```python
from build123d import *

# Parameters (mm, degrees)
F1_DEPTH = 26


with BuildPart() as f1:
    # F0 (on Top) → F1 (new body)
    with BuildSketch(Plane.XY):
        with BuildLine():
            ThreePointArc((-16.324504, 1), (-16.03161, 0.292893), (-15.324504, 0))
            Line((-15.324504, 0), (-0.324504, 0))
            ThreePointArc((-0.324504, 0), (0.382603, 0.292893), (0.675496, 1))
            ThreePointArc((0.675496, 1), (0.382603, 1.707107), (-0.324504, 2))
            Line((-0.324504, 2), (-13.324504, 2))
            ThreePointArc((-13.324504, 2), (-14.03161, 2.292893), (-14.324504, 3))
            Line((-14.324504, 3), (-14.324504, 8.393347))
            ThreePointArc((-14.324504, 8.393347), (-13.252645, 9.390761), (-12.334831, 8.25))
            Line((-12.334831, 8.25), (-0.564496, 8.25))
            Line((-0.564496, 8.25), (-0.564496, 8.948101))
            Line((-0.564496, 8.948101), (-0.564496, 9.25))
            ThreePointArc((-0.564496, 9.25), (-0.857389, 9.957107), (-1.564496, 10.25))
            Line((-1.564496, 10.25), (-15.324504, 10.25))
            ThreePointArc((-15.324504, 10.25), (-16.03161, 9.957107), (-16.324504, 9.25))
            Line((-16.324504, 9.25), (-16.324504, 1))
        make_face()
        with BuildLine():
            ThreePointArc((-12.334831, 8.25), (-13.252645, 9.390761), (-14.324504, 8.393347))
            Line((-14.324504, 8.393347), (-12.334831, 8.25))
        make_face()
    extrude(amount=F1_DEPTH)


solid = f1.part
```
Can you work these out from the model? Positions are in its coordinate system, mm. A direction names the side the tool comes from. Round coordinates to 2 decimals unless told otherwise and drop trailing zeros. Loops run counter-clockwise (first coordinate to the right, second up) from the corner with the lowest first, then second, coordinate; pieces in that order, holes last. Notation, with made-up numbers: (3.5, 24.5) -> (7.5, 24.5) arc R31 ccw to (7.5, 53.5) -> close; hole circle Ø1 at (45, 79). An arc over 180 degrees is marked (long way). One line per item, written item: value. Start each with the question number.
1. If we section it at D-D, the plane y = 6.5: Write out the boundary of the cut face in (x, z), then the cut area to 3 significant figures.
2. If we section it at A-A, the plane x = -12: Write out the boundary of the cut face in (y, z), then the cut area to 3 significant figures.
3. For pin 1 (1 mm diameter, centred on x = -13.5, y = 9, fed in from -Z); pin 2 (1.1 mm diameter, centred on y = 8.5, z = 15, fed in from +X); pin 3 (2.5 mm diameter, centred on y = 4.5, z = 18.5, fed in from +X), each with a flat end and sliding along its axis, tell me the tip position at first contact or that it passes through.
4. If we section it at C-C, the plane x = -1.25: Write out the boundary of the cut face in (y, z).
5. If I drill on probe 1 along Y at (x, z) = (-7, 17); probe 2 along X at (y, z) = (5, 24); probe 3 along Y at (x, z) = (-12.5, 6.75), over which ranges is the centre line in solid material (lowest first)?
6. If we section it at B-B, the plane z = 22.25: Write out the boundary of the cut face in (x, y).
7. For faces 1 (the flat face through (-7, 8.25, 13)), 2 (the cylindrical face through (-0.85, 9.95, 12.82)), 3 (the flat face through (-13.344, 8.323, 12.818)), which set-ups out of +Z, -Z, +X, -X, +Y, -Y let a thin tool reach every point of the face, with its end or its side?
8. If we mould it in two halves opening along Y, with no side actions, what happens to faces 4 (the flat face through (-7, 2, 13)), 5 (the flat face through (-0.564, 9, 13)), 6 (the cylindrical face through (-16.024, 9.965, 12.818))? For each: pulls with the +Y half, pulls with the -Y half, needs draft (parallel to the pull), parting line crosses it, or undercut.
Calculated:
1. outline: (-16.32, 0) -> (-14.32, 0) -> (-14.32, 26) -> (-16.32, 26) -> close
1. area: 52.0 mm²
2. outline: (0, 0) -> (2, 0) -> (2, 26) -> (0, 26) -> close; (8.25, 0) -> (10.25, 0) -> (10.25, 26) -> (8.25, 26) -> close
2. area: 104 mm²
3. pin 1: stops at z = 0
3. pin 2: stops at x = -0.56
3. pin 3: stops at x = -14.32
4. outline: (0, 0) -> (2, 0) -> (2, 26) -> (0, 26) -> close; (8.25, 0) -> (10.2, 0) -> (10.2, 26) -> (8.25, 26) -> close
5. probe 1: y = 0 to 2, 8.25 to 10.25
5. probe 2: x = -16.32 to -14.32
5. probe 3: y = 0 to 2, 8.26 to 10.25
6. outline: (-16.32, 1) arc R1 ccw to (-15.32, 0) -> (-0.32, 0) arc R1 ccw to (0.68, 1) arc R1 ccw to (-0.32, 2) -> (-13.32, 2) arc R1 cw to (-14.32, 3) -> (-14.32, 8.39) -> (-12.33, 8.25) -> (-0.56, 8.25) -> (-0.56, 9.25) arc R1 ccw to (-1.56, 10.25) -> (-15.32, 10.25) arc R1 ccw to (-16.32, 9.25) -> close
7. face 1: +Z, -Z, +X
7. face 2: +Z, -Z, +X, +Y
7. face 3: +Z, -Z
8. face 4: undercut
8. face 5: needs draft
8. face 6: pulls with the +Y half
